Source: CAD feature listing. Evaluate the final solid. Frame: model axes, mm. A direction names the side the tool comes from. Coordinates: 2 decimals unless noted, no trailing zeros. Order: outer loops, then holes, each group sorted by start corner. A loop starts at its lowest first (then second) coordinate and runs counter-clockwise, first axis right, second up.
Item 1: Mould query, pull axis Z, two halves, no side actions, for faces 6 (the flat face through (43, -1, 34)), 7 (the flat face through (-1, 1, -40)), 8 (the flat face through (-5, 1, 31)). Classes: released by +Z, released by -Z, zero draft, split by the parting line, or undercut.
Item 2: Reachability of faces 1 (the cylindrical face through (-48, 1, 39)), 2 (the flat face through (-5, 1, -31)), 3 (the flat face through (40, -1, 34.5)), 4 (the flat face through (40, -2, 36.5)), 5 (the flat face through (40.7, -2.4, -36.5)) from +Z, -Z, +X, -X, +Y, -Y: full face, straight path, thin tool, end or side. Return the list, or none.
Item 3: Section C-C on z = 0. Return the cut outline in (x, y), then the cut area to 4 significant figures.
Item 4: Section D-D on x = 46.4. Return the cut outline in (y, z), then the cut area to 3 significant figures.
Item 5: Section A-A on z = 24.5. Return the cut outline in (x, y), then the cut area to 3 significant figures.
Item 6: Ray query, line 1 (X direction, y = 1.4, z = 0); line 2 (Z direction, x = 8.5, y = 0.25); line 3 (Z direction, x = -46.4, y = 1.45). Return the intervals inside material, ascending.
Item 7: Section B-B on x = -17. Return the cut outline in (y, z), then the cut area to 4 significant figures.
Item 8: Contact query for flat-ended pins moving along their axis: P1, Ø8, axis at x = -28, z = -21, coming from the -Y side; P2, Ø2, axis at y = -2.5, z = -17, coming from the -X side; P3, Ø0.6, axis at y = -1.5, z = 34, coming from the +X side; P4, Ø1.6, axis at y = -1, z = -34, coming from the -X side. Output: stop coordinate, or through.
from build123d import *

# Parameters (mm, degrees)
SKETCH_1_R             = 1.35
SKETCH_1_W             = 51
SKETCH_1_H             = 65
EXTRUDE_1_DEPTH        = 3
SKETCH_2_W             = 6
SKETCH_2_H             = 4
EXTRUDE_2_DEPTH        = 4
SKETCH_4_R             = 1.15
CUT_EXTRUDE_2_DEPTH    = 4
FILLET_2_R             = 2
FILLET_2_OF_MIRROR_1_R = 2
SKETCH_5_R             = 3.75
CUT_EXTRUDE_3_DEPTH    = 3
EXTRUDE_3_DEPTH        = 1
SKETCH_7_R             = 1.15
EXTRUDE_4_DEPTH        = 2


with BuildPart() as part:
    # 草图1 → 凸台-拉伸1 (new body)
    with BuildSketch(Plane(origin=(0, 0, 0), x_dir=(1, 0, 0), z_dir=(0, 1, 0))):
        with BuildLine():
            Line((-45, 40), (45, 40))
            ThreePointArc((45, 40), (48.535533906, 38.535533906), (50, 35))
            Line((50, 35), (50, -35))
            ThreePointArc((50, -35), (48.535533906, -38.535533906), (45, -40))
            Line((45, -40), (-45, -40))
            ThreePointArc((-45, -40), (-48.535533906, -38.535533906), (-50, -35))
            Line((-50, -35), (-50, 35))
            ThreePointArc((-50, 35), (-48.535533906, 38.535533906), (-45, 40))
        make_face()
        with Locations((-46.4, 36.4)):
            Circle(SKETCH_1_R, mode=Mode.SUBTRACT)
        with Locations((46.4, 36.4)):
            Circle(SKETCH_1_R, mode=Mode.SUBTRACT)
        with Locations((46.4, -36.4)):
            Circle(SKETCH_1_R, mode=Mode.SUBTRACT)
        with Locations((-46.4, -36.4)):
            Circle(SKETCH_1_R, mode=Mode.SUBTRACT)
        with Locations((18.5, 0)):
            Rectangle(SKETCH_1_W, SKETCH_1_H, mode=Mode.SUBTRACT)
    extrude(amount=EXTRUDE_1_DEPTH)

    # 草图2 → 凸台-拉伸2 (add)
    with BuildSketch(Plane(origin=(0, 0, 0), x_dir=(-1, 0, 0), z_dir=(0, -1, 0))):
        with Locations((-40, 34.5)):
            Rectangle(SKETCH_2_W, SKETCH_2_H)
    extrude_2 = extrude(amount=EXTRUDE_2_DEPTH)

    # 草图4 → 切除-拉伸2 (cut)
    with BuildSketch(Plane.XY.offset(-32.5)):
        with Locations((40, -1.3)):
            Circle(SKETCH_4_R)
    cut_extrude_2 = extrude(amount=-CUT_EXTRUDE_2_DEPTH, mode=Mode.SUBTRACT)

    # 圆角2
    fillet_2_edges = [part.edges().sort_by_distance(p)[0] for p in [
        (43, -4, -34.5),
        (37, -4, -34.5),
    ]]
    fillet(fillet_2_edges, radius=FILLET_2_R)

    # 镜向1: 凸台-拉伸2, 切除-拉伸2 across plane
    add(extrude_2.mirror(Plane.XY))
    add(cut_extrude_2.mirror(Plane.XY), mode=Mode.SUBTRACT)

    # 圆角2 of 镜向1
    fillet_2_of_mirror_1_edges = [part.edges().sort_by_distance(p)[0] for p in [
        (43, -4, 34.5),
        (37, -4, 34.5),
    ]]
    fillet(fillet_2_of_mirror_1_edges, radius=FILLET_2_OF_MIRROR_1_R)

    # 草图5 → 切除-拉伸3 (cut)
    with BuildSketch(Plane(origin=(0, 3, 0), x_dir=(1, 0, 0), z_dir=(0, 1, 0))):
        with Locations((-17, 0)):
            Circle(SKETCH_5_R)
    extrude(amount=-CUT_EXTRUDE_3_DEPTH, mode=Mode.SUBTRACT)

    # 草图6 → 凸台-拉伸3 (add)
    with BuildSketch(Plane.XZ):
        with BuildLine():
            Line((-7, -28.5), (-7, -32.5))
            Line((-7, -32.5), (-3, -32.5))
            ThreePointArc((-3, -32.5), (-4.171572875, -29.671572875), (-7, -28.5))
        make_face()
        with BuildLine():
            Line((-7, 28.5), (-7, 32.5))
            Line((-7, 32.5), (-3, 32.5))
            ThreePointArc((-3, 32.5), (-4.171572875, 29.671572875), (-7, 28.5))
        make_face()
    extrude(amount=-EXTRUDE_3_DEPTH)

    # 草图7 → 凸台-拉伸4 (add)
    with BuildSketch(Plane.XY.offset(36.5)):
        with Locations((40, -1.3)):
            Circle(SKETCH_7_R)
    extrude(amount=-EXTRUDE_4_DEPTH)


solid = part.part
Answer list:
1. face 6: zero draft
1. face 7: released by -Z
1. face 8: undercut
2. face 1: +Z, -X, +Y, -Y
2. face 2: +Y
2. face 3: -Z
2. face 4: +Z, +X, -X, -Y
2. face 5: -Z, +X, -X, -Y
3. outline: (-50, 0) - (-20.75, 0) - (-20.75, 3) - (-50, 3) - close; (-13.25, 0) - (-7, 0) - (-7, 3) - (-13.25, 3) - close; (44, 0) - (50, 0) - (50, 3) - (44, 3) - close
3. area: 124.5 mm2
4. outline: (0, -39.8) - (3, -39.8) - (3, -37.75) - (0, -37.75) - close; (0, -35.05) - (3, -35.05) - (3, 35.05) - (0, 35.05) - close; (0, 37.75) - (3, 37.75) - (3, 39.8) - (0, 39.8) - close
4. area: 223 mm2
5. outline: (-50, 0) - (-7, 0) - (-7, 3) - (-50, 3) - close; (44, 0) - (50, 0) - (50, 3) - (44, 3) - close
5. area: 147 mm2
6. line 1: x = -50 to -20.75, -13.25 to -7, 44 to 50
6. line 2: z = -40 to -32.5, 32.5 to 40
6. line 3: z = -39.8 to -37.75, -35.05 to 35.05, 37.75 to 39.8
7. outline: (0, -40) - (3, -40) - (3, -3.75) - (0, -3.75) - close; (0, 3.75) - (3, 3.75) - (3, 40) - (0, 40) - close
7. area: 217.5 mm2
8. P1: stops at y = 0
8. P2: passes through
8. P3: stops at x = 43
8. P4: stops at x = 37
